Can you work these out from the model? Positions are in its coordinate system, mm. Face numbers are marked on the shaded views. A direction names the side the tool comes from. Round coordinates to 2 decimals unless told otherwise and drop trailing zeros. Write each loop counter-clockwise with the first axis right and the second up, starting at its lowest first coordinate (ties: lowest second). Pieces come first, ordered by that corner, then holes. Notation, with made-up numbers: (45, 11.5) - (95, 11.5) arc R27 ccw to (95, 41.5) - close; hole circle Ø10 at (85, 21.25). An arc over 180 degrees is marked (long way). One line per item, written item: value. Start each with the question number.
(1) I'm going to push flat-ended pins straight in: pin 1 Ø1.1 at (x, y) = (-17.5, 2.5) entering from -Z; pin 2 Ø1 at (x, y) = (17, 2.5) entering from -Z; pin 3 Ø3 at (y, z) = (2.5, 27.5) entering from -X. Where does each tip first touch, or does it pass through?
(2) If I drill on L1, parallel to X at y = 3.25, z = 3.5; L2, parallel to X at y = 3, z = 1.5; L3, parallel to Z at x = -2, y = 2, over which ranges is the centre line in solid material (lowest first)? Write a range as from..to.
(3) On a 3-axis mill with a long thin cutter (end or side, diameter ignored), from which of +Z, -Z, +X, -X, +Y, -Y can I reach the whole of each face in a straight line? I mean the marked faces 1 and 2. Say none if no direction works.
(4) I want a section at A-A on x = -10. List the corners of the cut face in (y, z) for me.
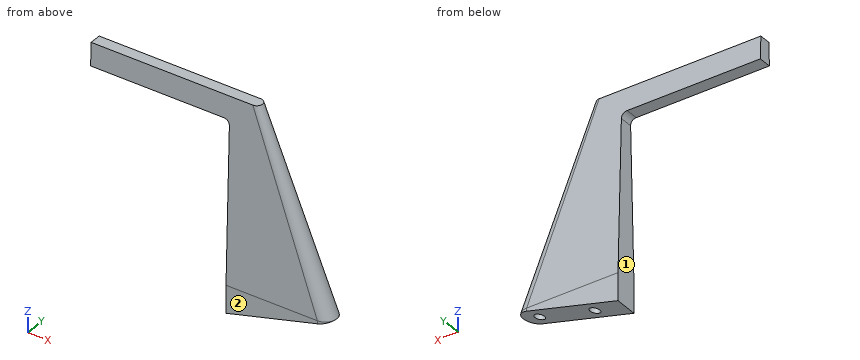
Autodesk Inventor part; units mm, degrees
ref_plane "Work Plane1" through (0, 0, 50.8) normal (0, 0, 1) x (1, 0, 0)
ref_plane "YZ Plane" through (0, 0, 0) normal (1, 0, 0) x (0, 1, 0)
ref_plane "XZ Plane" through (0, 0, 0) normal (0, 1, 0) x (-1, 0, 0)
sketch "Sketch2" plane through (0, 0, 0) normal (0, 0, 1) x (1, 0, 0)
  line L0 (0, 0) -> (25.4, 0)
  line L1 (25.4, 0) -> (25.4, 6.35)
  line L2 (25.4, 6.35) -> (0, 6.35)
  line L3 (0, 6.35) -> (0, 0)
  arc A0 (25.4, 0) -> (25.4, 6.35) centre (25.4, 3.175) ccw
  dimension "d0" = 25.4
  dimension "d1" = 6.35
ref_plane "Work Plane1" through (0, 0, 50.8) normal (0, 0, 1) x (1, 0, 0)
sketch "Sketch3" plane through (0, 0, 50.8) normal (0, 0, 1) x (1, 0, 0)
  line L0 (0, 1.5875) -> (6.35, 1.5875)
  line L1 (6.35, 1.5875) -> (6.35, 4.7625)
  line L2 (6.35, 4.7625) -> (0, 4.7625)
  line L3 (0, 4.7625) -> (0, 1.5875)
  arc A0 (6.35, 1.5875) -> (6.35, 4.7625) centre (6.35, 3.175) ccw
  point P0 (0, 0)
  dimension "d3" = 6.35
  dimension "d4" = 3.175
  dimension "d5" = 1.5875
loft "Loft1" add profiles "Sketch2", "Sketch3"
sketch "Sketch4" plane through (0, 0, 0) normal (-1, 0, 0) x (0, 0, 1)
  line L0 (0, 6.35) -> (0, 0)
  line L1 (0, 0) -> (50.8, 1.5875)
  line L2 (50.8, 4.7625) -> (50.8, 1.5875)
  line L3 (0, 6.35) -> (50.8, 4.7625)
  line L4 (0, 6.35) -> (50.8, 4.7625)
  line L5 (44.45, 4.960938) -> (44.45, 1.389063)
  line L6 (50.8, 1.5875) -> (0, 0)
  dimension "d10" = 6.35
extrude "Extrusion1" add sketch "Sketch4" along normal blind 38.608 contours L3 L2 L1 L5
sketch "Sketch5" plane through (25.4, 6.35, 0) normal (0, 0, -1) x (-1, 0, 0)
  line L0 (25.4, 0) -> (25.4, -6.35)
  line L1 (0, 0) -> (25.4, 0)
  arc A0 (0, 0) -> (0, -6.35) centre (0, -3.175) ccw
  line L2 (25.4, -6.35) -> (0, -6.35)
  line L3 (25.4, 0) -> (25.4, -6.35)
  line L4 (25.4, 0) -> (36.148692, 0)
  line L5 (36.148692, 0) -> (36.148692, -6.35)
  line L6 (36.148692, -6.35) -> (25.4, -6.35)
  line L7 (25.4, -6.35) -> (25.4, 0)
  line L8 (-3.175, -0.10761) -> (-3.175, -7.006989)
sketch "Sketch5 outline for Revolution1" plane through (25.4, 6.35, 0) normal (0, 0, -1) x (-1, 0, 0)
  line L0 (36.148692, 0) -> (0, 0)
  arc A0 (0, 0) -> (0, -6.35) centre (0, -3.175) ccw
  line L1 (0, -6.35) -> (36.148692, -6.35)
  line L2 (36.148692, -6.35) -> (36.148692, 0)
revolve "Revolution1" add sketch "Sketch5 outline for Revolution1" angle 15 about axis through (28.575, 6.24239, 0) along (0, -1, 0)
sketch "Sketch7" plane through (-10.748692, 6.35, 0) normal (0, 1, 0) x (1, 0, 0)
  line L0 (0, 0) -> (10.748692, 0)
  line L1 (36.148692, 0) -> (10.748692, 0)
  arc A0 (36.256878, 0.82175) -> (36.148692, 0) centre (39.323692, 0) ccw
  line L2 (1.339922, 10.17772) -> (36.256878, 0.82175)
  arc A1 (1.339922, 10.17772) -> (0, 0) centre (39.323692, 0) ccw
  line L3 (10.748692, 0) -> (10.748692, -44.45)
  line L4 (10.748692, 0) -> (-2.055619, 0)
  line L5 (-2.055619, 0) -> (-2.055619, 10.694673)
  line L6 (-2.055619, 10.694673) -> (10.748692, 10.694673)
  line L7 (10.748692, 10.694673) -> (10.748692, 0)
extrude "Extrusion2" cut sketch "Sketch7" against normal blind 38.1 contours A1 L2 L7 L0 | L4 L5 L6 L7 L2 A1
fillet "Fillet1" radius 1.5875 1 edges at (0, 3.175, 44.45)
sketch "Sketch8" plane through (0, 0, -7.656648) normal (0.258819, 0, -0.9659258) x (-0.9659258, 0, -0.258819)
  line L0 (-29.583017, 3.175) -> (-24.820517, 3.175)
  line L1 (-24.820517, 3.175) -> (-8.945517, 3.175)
  circle A0 centre (-24.820517, 3.175) radius 1.397
  circle A1 centre (-8.945517, 3.175) radius 1.397
  line L2 (-26.408017, 0) -> (0, 0)
  point P0 (-1.981686, 0)
  dimension "d17" = 4.7625
  dimension "d18" = 15.875
  dimension "d19" = 2.794
  dimension "d20" = 2.794
  dimension "d23" = 3.175
extrude "Extrusion4" cut sketch "Sketch8" against normal blind 12.7
properties part number "DivePlanesStabilizingFins"
Established:
1. pin 1: z = 44.45
1. pin 2: z = -3.24
1. pin 3: x = 0
2. L1: 0..4.83, 7.72..21.26, 24.15..27.15
2. L2: 0..5.37, 8.24..21.81, 24.68..27.96
2. L3: 44.45..50.8
3. face 1: -Z, -X, +Y, -Y
3. face 2: +Z, -Z, +X, -X, -Y
4. outline: (1.39, 44.45) - (4.96, 44.45) - (4.76, 50.8) - (1.59, 50.8) - close
